CAD build for the part. Positions are in the model's coordinates, mm. A direction names the side the tool comes from. Give positions to 0.01 mm unless a question says otherwise; leave off trailing zeros. Loops run counter-clockwise (first coordinate to the right, second up) from the corner with the lowest first, then second, coordinate; pieces in that order, holes last. Notation, with made-up numbers: M 68,8.25 L 79,8.25 A4 ccw 79,12.25 Z; hole C 11.5,-7.5 d2. An arc over 180 degrees is marked long. One line per question, with ' | ' between items.
```python
from build123d import *

# Parameters (mm, degrees)
ESQUISSE2_W                     = 57
ESQUISSE2_H                     = 57
BOSS_EXTRU_1_DEPTH              = 3.5
ESQUISSE3_W                     = 14.1
ESQUISSE3_H                     = 14.1
ENL_V_MAT_EXTRU_1_DEPTH         = 3.5
ESQUISSE4_W                     = 5
ESQUISSE4_H                     = 2
ENL_V_MAT_EXTRU_2_DEPTH         = 2
R_P_TITION_LIN_AIRE1_COUNT      = 3
R_P_TITION_LIN_AIRE1_PITCH      = 19
R_P_TITION_LIN_AIRE1_COUNT_DIR2 = 3
R_P_TITION_LIN_AIRE1_PITCH_DIR2 = 19


with BuildPart() as part:
    # Esquisse2 → Boss.-Extru.1 (new body)
    with BuildSketch(Plane(origin=(0, 0, 0), x_dir=(1, 0, 0), z_dir=(0, 1, 0))):
        Rectangle(ESQUISSE2_W, ESQUISSE2_H)
    extrude(amount=BOSS_EXTRU_1_DEPTH)

    # Esquisse3 → Enlèv. mat.-Extru.1 (cut)
    with BuildSketch(Plane(origin=(0, 3.5, 0), x_dir=(1, 0, 0), z_dir=(0, 1, 0))):
        with Locations((-18.95, 18.95)):
            Rectangle(ESQUISSE3_W, ESQUISSE3_H)
    enl_v_mat_extru_1 = extrude(amount=-ENL_V_MAT_EXTRU_1_DEPTH, mode=Mode.SUBTRACT)

    # Esquisse4 → Enlèv. mat.-Extru.2 (cut)
    with BuildSketch(Plane(origin=(0, 3.5, 0), x_dir=(1, 0, 0), z_dir=(0, 1, 0))):
        with Locations((-18.95, 26)):
            Rectangle(ESQUISSE4_W, ESQUISSE4_H)
        with Locations((-18.95, 11.9)):
            Rectangle(ESQUISSE4_W, ESQUISSE4_H)
    enl_v_mat_extru_2 = extrude(amount=-ENL_V_MAT_EXTRU_2_DEPTH, mode=Mode.SUBTRACT)

    # Répétition linéaire1: Enlèv. mat.-Extru.1, Enl_v. mat.-Extru.2 3 × 3
    with Locations(*[(i * R_P_TITION_LIN_AIRE1_PITCH, 0, j * R_P_TITION_LIN_AIRE1_PITCH_DIR2) for i in range(R_P_TITION_LIN_AIRE1_COUNT) for j in range(R_P_TITION_LIN_AIRE1_COUNT_DIR2) if (i, j) != (0, 0)]):
        add(enl_v_mat_extru_1, mode=Mode.SUBTRACT)
        add(enl_v_mat_extru_2, mode=Mode.SUBTRACT)


solid = part.part
```
Item 1: Saw through at C-C on y = 0.9. State how many separate pieces and enclosed holes the cut face has, and give its area (3 significant figures).
Conclusion:
separate pieces: 1 | enclosed holes: 9 | area: 1,460 mm²
Item 2: Drill centre lines: line 1 along Z through (x, y) = (-17.5, 1.15); line 2 along Z through (x, y) = (-21, 1.7). Where is each one in solid material? Low to high. Write a range as [from, to].
Conclusion:
line 1: [-28.5, -26], [-11.9, -7], [7.1, 12], [26.1, 28.5] | line 2: [-28.5, -27], [-10.9, -8], [8.1, 11], [27.1, 28.5]
Item 3: Saw through at B-B on x = -20. Give the cut face in (y, z), and give its area (4 significant figures).
Conclusion:
outline: M 0,-28.5 L 3.5,-28.5 L 3.5,-27 L 1.5,-27 L 1.5,-26 L 0,-26 Z; M 0,-11.9 L 1.5,-11.9 L 1.5,-10.9 L 3.5,-10.9 L 3.5,-8 L 1.5,-8 L 1.5,-7 L 0,-7 Z; M 0,7.1 L 1.5,7.1 L 1.5,8.1 L 3.5,8.1 L 3.5,11 L 1.5,11 L 1.5,12 L 0,12 Z; M 0,26.1 L 1.5,26.1 L 1.5,27.1 L 3.5,27.1 L 3.5,28.5 L 0,28.5 Z | area: 39.45 mm²
Item 4: Saw through at A-A on z = 2. Give the cut face in (x, y), and give its area (4 significant figures).
Conclusion:
outline: M -28.5,0 L -26,0 L -26,3.5 L -28.5,3.5 Z; M -11.9,0 L -7,0 L -7,3.5 L -11.9,3.5 Z; M 7.1,0 L 12,0 L 12,3.5 L 7.1,3.5 Z; M 26.1,0 L 28.5,0 L 28.5,3.5 L 26.1,3.5 Z | area: 51.45 mm²
Item 5: Drop flat-ended pins along their axis: P1, Ø1.1, axis at x = 0, z = 7.5, coming from the +Y side; P2, Ø1.5, axis at x = 17.5, z = -7.5, coming from the +Y side. Give the stop position or say it passes through.
Conclusion:
P1: y = 1.5 | P2: y = 3.5
Item 6: 3-axis set-ups, long thin cutter, end or side, ignore diameter. For faces 1 (the flat face through (0, 2, -28.5)), 2 (the flat face through (0, 3, -8)), 3 (the flat face through (0, 1, 7.1)): which of +Z, -Z, +X, -X, +Y, -Y reach the whole face in a straight line?
Conclusion:
face 1: -Z, +X, -X, +Y, -Y | face 2: +Y | face 3: +Y, -Y
